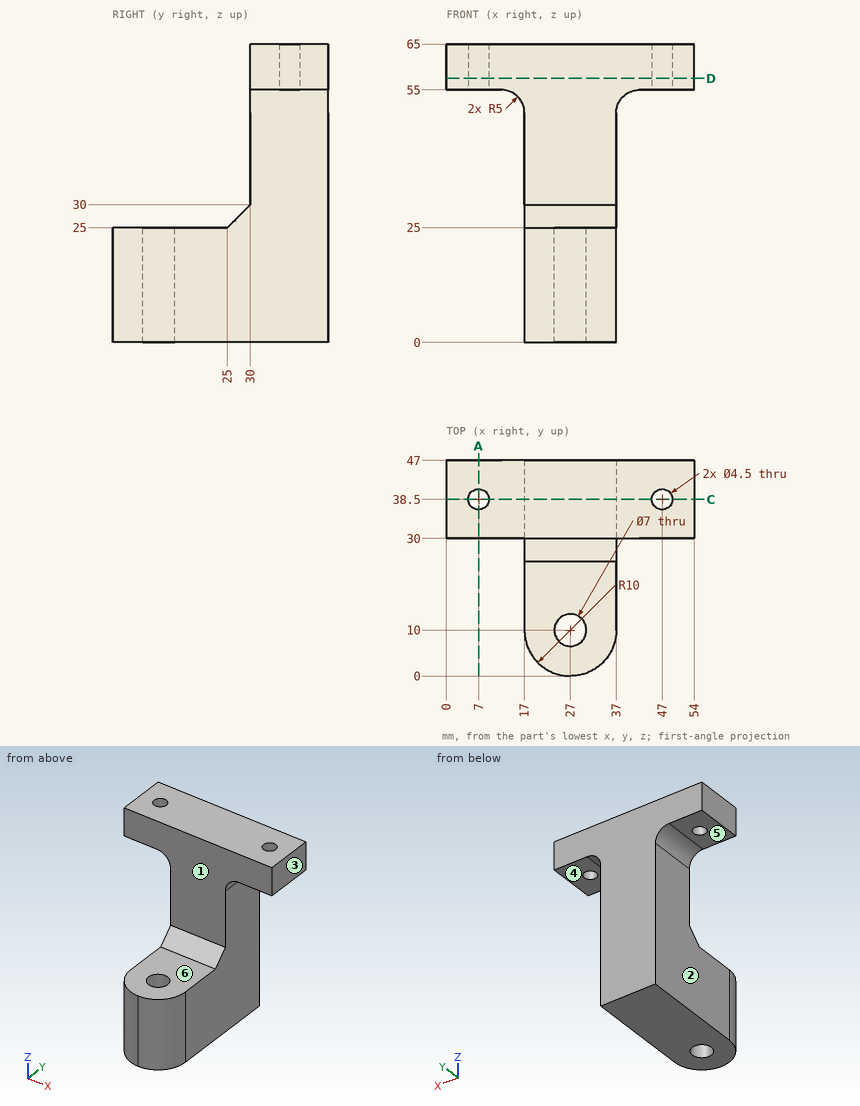
The drawing under review shows one solid part. Ordinate dimensions are in mm from its lowest x, y, z. A direction names the side the tool comes from. Round coordinates to 2 decimals unless told otherwise and drop trailing zeros. Loops run counter-clockwise (first coordinate to the right, second up) from the corner with the lowest first, then second, coordinate; pieces in that order, holes last.
Item 1: For the marked faces 4, 5 and 6, list the 3-axis set-ups (+Z, -Z, +X, -X, +Y, -Y) from which the entire face can be reached by the end or side of a thin tool; tool diameter is ignored.
Determined:
face 4: -Z, +X, +Y, -Y
face 5: -Z, -X, +Y, -Y
face 6: +Z, +X, -X, -Y
Item 2: Take a section at C-C (y = 38.5). Write out the cut boundary in (x, z).
Determined:
outline: (0, 55) - (4.75, 55) - (4.75, 65) - (0, 65) - close; (9.25, 55) - (12, 55) arc R5 cw to (17, 50) - (17, 0) - (37, 0) - (37, 50) arc R5 cw to (42, 55) - (44.75, 55) - (44.75, 65) - (9.25, 65) - close; (49.25, 55) - (54, 55) - (54, 65) - (49.25, 65) - close
Item 3: Take a section at D-D (z = 57.5). Write out the cut boundary in (x, y), then the cut area to 3 significant figures.
Determined:
outline: (0, 30) - (54, 30) - (54, 47) - (0, 47) - close; hole circle Ø4.5 at (7, 38.5); hole circle Ø4.5 at (47, 38.5)
area: 886 mm2
Item 4: Take a section at A-A (x = 7). Write out the cut boundary in (y, z), then the cut area to 3 significant figures.
Determined:
outline: (30, 55) - (36.25, 55) - (36.25, 65) - (30, 65) - close; (40.75, 55) - (47, 55) - (47, 65) - (40.75, 65) - close
area: 125 mm2
Item 5: For line 1 (Y direction, x = 47, z = 60.5); line 2 (Y direction, x = 27, z = 13); line 3 (Z direction, x = 31.5, y = 21.5), list the stretches that pass through material, from the lowest coordinate up.
Determined:
line 1: y = 30 to 36.25, 40.75 to 47
line 2: y = 0 to 6.5, 13.5 to 47
line 3: z = 0 to 25
Item 6: Mouldability with a two-part tool opening along X and no side actions: class the marked faces 1, 2 and 3 as released by +X, released by -X, zero draft, split by the parting line, or undercut.
Determined:
face 1: zero draft
face 2: released by -X
face 3: released by +X
Item 7: Clearance check with flat-ended pins moving along their axes: pin 1 Ø2 at (x, z) = (30, 38) entering from -Y; pin 2 Ø5 at (x, y) = (7, 38.5) entering from +Z; pin 3 Ø13 at (x, y) = (48, 35.5) entering from -Z; pin 4 Ø11 at (x, y) = (27, 10) entering from +Z. State where each tip first meets the part, or that it passes through.
Determined:
pin 1: stops at y = 30
pin 2: stops at z = 65
pin 3: stops at z = 54.97
pin 4: stops at z = 25
